```python
from build123d import *

# Parameters (mm, degrees)
SKETCH1_W           = 100
SKETCH1_H           = 250
BOSS_EXTRUDE1_DEPTH = 100
SKETCH2_W           = 50
SKETCH2_H           = 5
SKETCH2_W_2         = 5
SKETCH2_H_2         = 50
BOSS_EXTRUDE2_DEPTH = 250
FILLET3_R           = 2.5
FILLET4_R           = 2.5


with BuildPart() as part:
    # Sketch1 → Boss-Extrude1 (new body)
    with BuildSketch(Plane(origin=(0, 0, 0), x_dir=(1, 0, 0), z_dir=(0, 1, 0))):
        with Locations((50, 125)):
            Rectangle(SKETCH1_W, SKETCH1_H)
    extrude(amount=BOSS_EXTRUDE1_DEPTH)

    # Sketch2 → Boss-Extrude2 (add)
    with BuildSketch(Plane.XY):
        with Locations((125, 87.5)):
            Rectangle(SKETCH2_W, SKETCH2_H)
        with Locations((125, 97.5)):
            Rectangle(SKETCH2_W, SKETCH2_H)
        with Locations((125, 77.5)):
            Rectangle(SKETCH2_W, SKETCH2_H)
        with Locations((125, 67.5)):
            Rectangle(SKETCH2_W, SKETCH2_H)
        with Locations((17.5, 125)):
            Rectangle(SKETCH2_W_2, SKETCH2_H_2)
        with Locations((7.5, 125)):
            Rectangle(SKETCH2_W_2, SKETCH2_H_2)
        with Locations((27.5, 125)):
            Rectangle(SKETCH2_W_2, SKETCH2_H_2)
        with Locations((37.5, 125)):
            Rectangle(SKETCH2_W_2, SKETCH2_H_2)
        with Locations((47.5, 125)):
            Rectangle(SKETCH2_W_2, SKETCH2_H_2)
        with Locations((57.5, 125)):
            Rectangle(SKETCH2_W_2, SKETCH2_H_2)
        with Locations((67.5, 125)):
            Rectangle(SKETCH2_W_2, SKETCH2_H_2)
        with Locations((77.5, 125)):
            Rectangle(SKETCH2_W_2, SKETCH2_H_2)
        with Locations((87.5, 125)):
            Rectangle(SKETCH2_W_2, SKETCH2_H_2)
        with Locations((125, 25)):
            Rectangle(SKETCH2_W, SKETCH2_H_2)
        with Locations((125, 57.5)):
            Rectangle(SKETCH2_W, SKETCH2_H)
    extrude(amount=-BOSS_EXTRUDE2_DEPTH)

    # Fillet3
    fillet3_edges = [part.edges().sort_by_distance(p)[0] for p in [
        (80, 100, -125),
        (75, 100, -125),
        (90, 100, -125),
        (85, 100, -125),
        (5, 100, -125),
        (10, 100, -125),
        (20, 100, -125),
        (15, 100, -125),
        (30, 100, -125),
        (25, 100, -125),
        (40, 100, -125),
        (35, 100, -125),
        (50, 100, -125),
        (45, 100, -125),
        (60, 100, -125),
        (55, 100, -125),
        (70, 100, -125),
        (65, 100, -125),
    ]]
    fillet(fillet3_edges, radius=FILLET3_R - 0.0001)  # a hair under: the kernel refuses the full size

    # Fillet4
    fillet4_edges = [part.edges().sort_by_distance(p)[0] for p in [
        (100, 55, -125),
        (100, 65, -125),
        (100, 75, -125),
        (100, 85, -125),
        (100, 95, -125),
        (100, 90, -125),
        (100, 80, -125),
        (100, 70, -125),
        (100, 60, -125),
        (100, 50, -125),
    ]]
    fillet(fillet4_edges, radius=FILLET4_R - 0.0001)  # a hair under: the kernel refuses the full size


solid = part.part
```
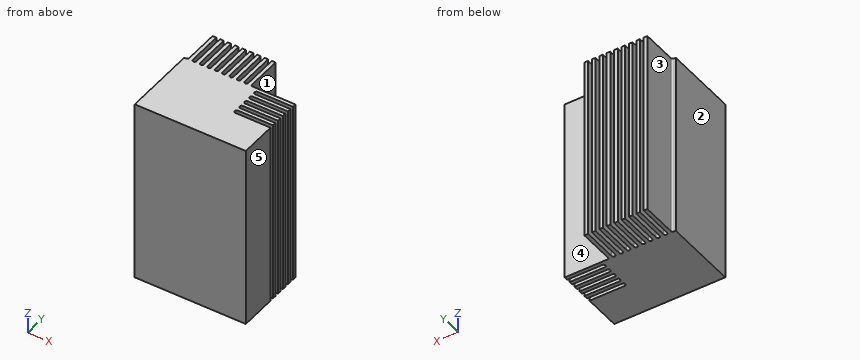
Source: CAD feature listing. Evaluate the final solid. Frame: model axes, mm. Face numbers are marked on the shaded views. A direction names the side the tool comes from. Coordinates: 2 decimals unless noted, no trailing zeros. Loops run counter-clockwise (first coordinate to the right, second up) from the corner with the lowest first, then second, coordinate; pieces in that order, holes last. Notation, with made-up numbers: (-15.75, -32) -> (31.25, -32) arc R12 ccw to (31.25, -11) -> close; hole circle Ø10 at (62.5, 21.5). An arc over 180 degrees is marked (long way). One line per item, written item: value. Start each with the question number.
Q1. Set-up query: the marked faces 1 and 2. Return all of +Z, -Z, +X, -X, +Y, -Y with unobstructed straight access to the full face (end or side cutting, diameter ignored); none if empty.
Q2. Contact query for flat-ended pins moving along their axis: P1, Ø24, axis at y = 120.5, z = -87.5, coming from the -X side; P2, Ø1.5, axis at y = 115.5, z = -99, coming from the +X side; P3, Ø14.5, axis at x = 125.5, z = -149.5, coming from the +Y side. Output: stop coordinate, or through.
Q3. Section query B-B, the plane y = 122. Give the number of separate pieces and of enclosed holes in the cut face, and give its area (4 significant figures).
Q4. Line query: line 1 along Y through (x, z) = (120, -95); line 2 along Y through (x, z) = (100.5, -129); line 3 along Y through (x, z) = (43, -107). Output: solid intervals per line, ascending.
Q5. Mould query, pull axis X, two halves, no side actions, for the marked faces 3, 4 and 5. Classes: pulls with the +X half, pulls with the -X half, needs draft (parallel to the pull), parting line crosses it, or undercut.
Q6. Section query A-A, the plane x = 131.5. Return the cut outline in (y, z).
Results:
1. face 1: +Z, -Z, +X, +Y
1. face 2: +Z, -Z, -X, +Y, -Y
2. P1: x = 5
2. P2: x = 90
2. P3: y = 100
3. separate pieces: 9
3. enclosed holes: 0
3. area: 11,250 mm^2
4. line 1: 0 to 50, 55 to 60, 65 to 70, 75 to 80, 85 to 90, 95 to 100
4. line 2: 0 to 51, 54 to 61, 64 to 71, 74 to 81, 84 to 91, 94 to 100
4. line 3: 0 to 100.05
5. face 3: pulls with the -X half
5. face 4: needs draft
5. face 5: pulls with the +X half
6. outline: (0, -250) -> (50, -250) -> (50, 0) -> (0, 0) -> close; (55, -250) -> (60, -250) -> (60, 0) -> (55, 0) -> close; (65, -250) -> (70, -250) -> (70, 0) -> (65, 0) -> close; (75, -250) -> (80, -250) -> (80, 0) -> (75, 0) -> close; (85, -250) -> (90, -250) -> (90, 0) -> (85, 0) -> close; (95, -250) -> (100, -250) -> (100, 0) -> (95, 0) -> close
